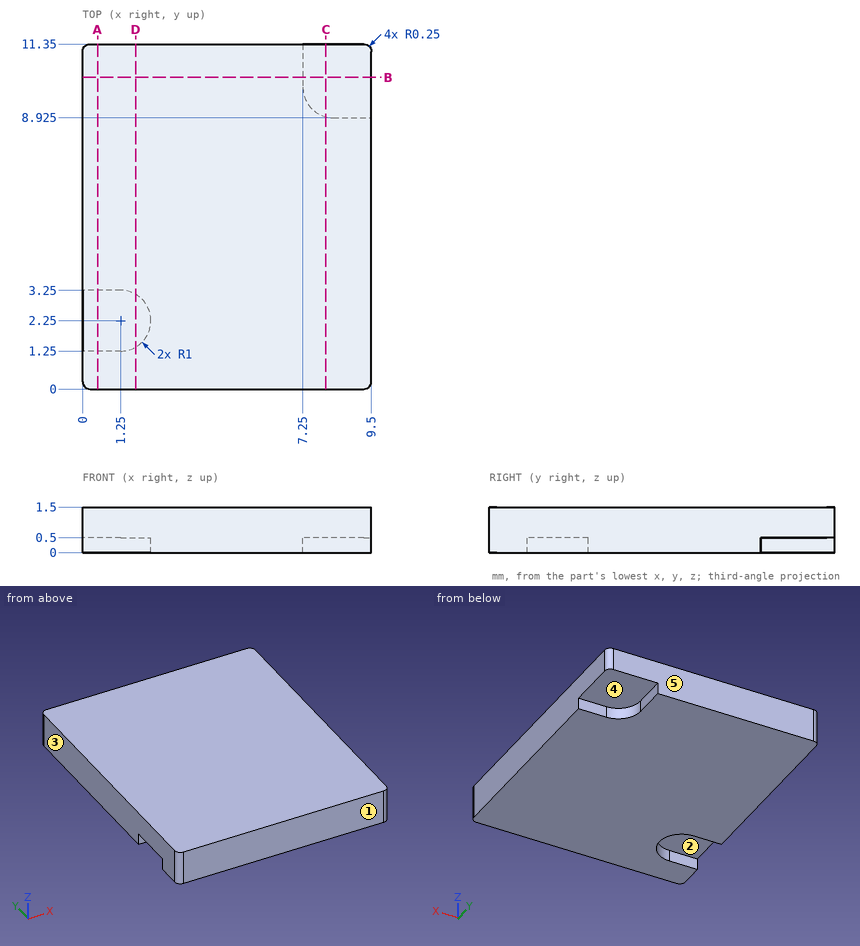
Geometry: see drawing. Coordinates: mm, zero at the bounding-box minimum. A direction names the side the tool comes from. Round coordinates to 2 decimals unless told otherwise and drop trailing zeros. Write each loop counter-clockwise with the first axis right and the second up, starting at its lowest first coordinate (ties: lowest second). Pieces come first, ordered by that corner, then holes. Notation, with made-up numbers: (80.25, 26) - (132.25, 26) arc R25 ccw to (132.25, 60) - close; hole circle Ø4 at (16, 61). An arc over 180 degrees is marked (long way). Use CSV: the item, a comma, the result in double quotes. Start each with the question number.
(1) Cut plane B-B, the plane y = 10.25. Return loops of the section in (x, z), and give its area (3 significant figures).
(2) Cut plane D-D, the plane x = 1.75. Return loops of the section in (y, z).
(3) Cut plane A-A, the plane x = 0.5. Return loops of the section in (y, z).
(4) Material intervals for probe 1 along Y at (x, z) = (1, 0.4); probe 2 along Z at (x, y) = (8.5, 9.25); probe 3 along X at (y, z) = (9.25, 0.4), sorted ascending. Write a range as [from, to].
(5) Mould query, pull axis Y, two halves, no side actions, for the marked faces 1, 2 and 3. Classes: pulls with the +Y half, pulls with the -Y half, needs draft (parallel to the pull), parting line crosses it, or undercut.
(6) Set-up query: the marked faces 4 and 5. Return all of +Z, -Z, +X, -X, +Y, -Y with unobstructed straight access to the full face (end or side cutting, diameter ignored); none if empty.
(7) First-contact query: pin 1 Ø0.7 at (x, y) = (8.5, 10.5) entering from -Z. Flat tip, straight axial feed; report the tip coordinate or a pass-through.
(8) Cut plane C-C, the plane x = 8. Return loops of the section in (y, z), and give its area (3 significant figures).
Geometry says:
1,outline,"(0, 0) - (7.25, 0) - (7.25, 0.5) - (9.5, 0.5) - (9.5, 1.5) - (0, 1.5) - close"
1,area,"13.1 mm²"
2,outline,"(0, 0) - (1.38, 0) - (1.38, 0.5) - (3.12, 0.5) - (3.12, 0) - (11.35, 0) - (11.35, 1.5) - (0, 1.5) - close"
3,outline,"(0, 0) - (1.25, 0) - (1.25, 0.5) - (3.25, 0.5) - (3.25, 0) - (11.35, 0) - (11.35, 1.5) - (0, 1.5) - close"
4,probe 1,"[0, 1.25], [3.25, 11.35]"
4,probe 2,"[0.5, 1.5]"
4,probe 3,"[0, 7.51]"
5,face 1,"pulls with the -Y half"
5,face 2,"undercut"
5,face 3,"needs draft"
6,face 4,"-Z, +X, +Y"
6,face 5,"+Z, -Z, +X, -X, +Y"
7,pin 1,"z = 0.5"
8,outline,"(0, 0) - (8.96, 0) - (8.96, 0.5) - (11.35, 0.5) - (11.35, 1.5) - (0, 1.5) - close"
8,area,"15.8 mm²"
